Read the model definition and answer for the solid it produces. Units are mm, in the model's axes. A direction names the side the tool comes from. Give positions to 0.01 mm unless a question says otherwise; leave off trailing zeros. Write each loop counter-clockwise with the first axis right and the second up, starting at its lowest first coordinate (ties: lowest second). Pieces come first, ordered by that corner, then holes. Notation, with made-up numbers: M 60,1 L 109,1 A13 ccw 109,20 Z; hole C 70.25,-32.5 d9. An arc over 180 degrees is marked long. Put each result on its own line as item: value.
from build123d import *

# Parameters (mm, degrees)
F1_DEPTH  = 150
F2_T      = -2
F4_W      = 121
F4_H      = 42
F5_DEPTH  = 3
F6_R      = 3
F8_R      = 1.5
F8_R_2    = 0.75
F9_DEPTH  = 8.5
F10_R     = 2.5
F10_R_2   = 1.5
F12_R     = 2.5
F12_R_2   = 1.25
F13_REACH = 69.4690374315
F14_W     = 150
F14_H     = 127.2792206136
F14_W_2   = 146
F14_H_2   = 121.6223663641
F15_DEPTH = 2.5
F16_R     = 2.5
F16_R_2   = 1.25
F18_R     = 2
F19_R     = 0.5
F7_W      = 10
F7_H      = 12
F7_W_2    = 13.1
F7_H_2    = 11.7
F20_DEPTH = 3
F21_R     = 0.5
F22_R     = 0.5
F23_R     = 6.5
F24_DEPTH = 2.5
F25_R     = 2.5
F25_R_2   = 1.25
F26_DEPTH = 2.5
F27_R     = 2.5
F28_DEPTH = 1.5
F29_R     = 3


with BuildPart() as f1:
    # F0 (on Right) → F1 (new body)
    with BuildSketch(Plane.YZ):
        Polygon((63.6396103068, 63.6396103068), (0, 0), (127.2792206136, 0), align=None)
    extrude(amount=F1_DEPTH)

    # F2
    f2_openings = [f1.faces().sort_by_distance(p)[0] for p in [
        (75, 63.63961, 0),
    ]]
    offset(amount=F2_T, openings=f2_openings)

    # F4 (on offset) → F5 (cut)
    with BuildSketch(Plane(origin=(0, 0, 0), x_dir=(1, 0, 0), z_dir=(0, -0.7071067812, 0.7071067812))):
        with Locations((75, 45)):
            Rectangle(F4_W, F4_H)
    extrude(amount=-F5_DEPTH, mode=Mode.SUBTRACT)

    # F6
    f6_edges = [f1.edges().sort_by_distance(p)[0] for p in [
        (75, 63.63961, 63.63961),
    ]]
    fillet(f6_edges, radius=F6_R)

    # F8 (on face) → F9 (join)
    with BuildSketch(Plane(origin=(0, 0, 0), x_dir=(1, 0, 0), z_dir=(0, -0.7071067812, 0.7071067812))):
        with Locations((131, 67.5)):
            Circle(F8_R)
        with Locations((131, 67.5)):
            Circle(F8_R_2, mode=Mode.SUBTRACT)
        with Locations((131, 22.5)):
            Circle(F8_R)
        with Locations((131, 22.5)):
            Circle(F8_R_2, mode=Mode.SUBTRACT)
        with Locations((19, 67.5)):
            Circle(F8_R)
        with Locations((19, 67.5)):
            Circle(F8_R_2, mode=Mode.SUBTRACT)
        with Locations((19, 22.5)):
            Circle(F8_R)
        with Locations((19, 22.5)):
            Circle(F8_R_2, mode=Mode.SUBTRACT)
    extrude(amount=-F9_DEPTH)

    # F10 (on face) → F11 (join, up to the last surface of F1)
    with BuildSketch(Plane(origin=(0, 0, 0), x_dir=(1, 0, 0), z_dir=(0, 0, -1))):
        with Locations((10, -10)):
            Circle(F10_R)
        with Locations((10, -10)):
            Circle(F10_R_2, mode=Mode.SUBTRACT)
    extrude(until=Until.LAST, dir=(0, 0, 1))

    f13_end = Plane(origin=(75.2433178079, 33.3209918004, 30.4925646757), x_dir=(0, 0.7071067812, 0.7071067812), z_dir=(0, 0.7071067812, -0.7071067812))
    # F12 (on face) → F13 (join, up to a plane its end follows)
    with BuildSketch(Plane(origin=(0, 0, 0), x_dir=(1, 0, 0), z_dir=(0, 0, -1))):
        with Locations((10, -10)):
            Circle(F12_R)
        with Locations((10, -10)):
            Circle(F12_R_2, mode=Mode.SUBTRACT)
        with Locations((140, -10)):
            Circle(F12_R)
        with Locations((140, -10)):
            Circle(F12_R_2, mode=Mode.SUBTRACT)
    f13_long = extrude(amount=-F13_REACH, mode=Mode.PRIVATE)
    add(split(f13_long, bisect_by=f13_end, keep=Keep.TOP, mode=Mode.PRIVATE))

    # F14 (on face) → F15 (join)
    with BuildSketch(Plane(origin=(0, 0, 0), x_dir=(1, 0, 0), z_dir=(0, 0, -1))):
        with Locations((75, -63.6396103068)):
            Rectangle(F14_W, F14_H)
        with Locations((75, -63.6396103068)):
            Rectangle(F14_W_2, F14_H_2, mode=Mode.SUBTRACT)
    extrude(amount=F15_DEPTH)

    # F16 (on Top) → F17 (join, up to the next surface of F1)
    with BuildSketch(Plane.XY):
        with Locations((140, 117.279)):
            Circle(F16_R)
        with Locations((140, 117.279)):
            Circle(F16_R_2, mode=Mode.SUBTRACT)
        with Locations((10, 117.279)):
            Circle(F16_R)
        with Locations((10, 117.279)):
            Circle(F16_R_2, mode=Mode.SUBTRACT)
    extrude(until=Until.NEXT)

    # F18
    f18_edges = [f1.edges().sort_by_distance(p)[0] for p in [
        (150, 127.279221, -1.25),
        (150, 0, -1.25),
        (0, 0, -1.25),
        (0, 127.279221, -1.25),
    ]]
    fillet(f18_edges, radius=F18_R)

    # F19
    f19_edges = [f1.edges().sort_by_distance(p)[0] for p in [
        (0, 31.759145, 31.759145),
    ]]
    fillet(f19_edges, radius=F19_R)

    # F7 (on face) → F20 (cut)
    with BuildSketch(Plane.YZ.offset(150)):
        with Locations((95.7792206136, 10.65)):
            Rectangle(F7_W, F7_H)
        with Locations((65.3223664939, 10.0139604606)):
            Rectangle(F7_W_2, F7_H_2)
    extrude(amount=-F20_DEPTH, mode=Mode.SUBTRACT)

    # F21
    f21_edges = [f1.edges().sort_by_distance(p)[0] for p in [
        (149, 90.779221, 16.65),
        (149, 100.779221, 16.65),
    ]]
    fillet(f21_edges, radius=F21_R)

    # F22
    f22_edges = [f1.edges().sort_by_distance(p)[0] for p in [
        (149, 71.872366, 15.86396),
        (149, 58.772366, 15.86396),
    ]]
    fillet(f22_edges, radius=F22_R)

    # F23 (on face) → F24 (cut)
    with BuildSketch(Plane(origin=(0, 0, 0), x_dir=(0, -1, 0), z_dir=(-1, 0, 0))):
        with Locations((-64, 47.5)):
            Circle(F23_R)
    extrude(amount=-F24_DEPTH, mode=Mode.SUBTRACT)

    # F25 (on face) → F26 (join)
    with BuildSketch(Plane(origin=(0, 0, 0), x_dir=(1, 0, 0), z_dir=(0, 0, -1))):
        with Locations((10, -10)):
            Circle(F25_R)
        with Locations((10, -10)):
            Circle(F25_R_2, mode=Mode.SUBTRACT)
        with Locations((140, -10)):
            Circle(F25_R)
        with Locations((140, -10)):
            Circle(F25_R_2, mode=Mode.SUBTRACT)
        with Locations((10, -117.279)):
            Circle(F25_R)
        with Locations((10, -117.279)):
            Circle(F25_R_2, mode=Mode.SUBTRACT)
        with Locations((140, -117.279)):
            Circle(F25_R)
        with Locations((140, -117.279)):
            Circle(F25_R_2, mode=Mode.SUBTRACT)
    extrude(amount=F26_DEPTH)

    # F27 (on face) → F28 (cut)
    with BuildSketch(Plane(origin=(0, 0, 0), x_dir=(0, -1, 0), z_dir=(-1, 0, 0))):
        with Locations((-64, 32.5)):
            Circle(F27_R)
    extrude(amount=-F28_DEPTH, mode=Mode.SUBTRACT)

    # F29
    f29_edges = [f1.edges().sort_by_distance(p)[0] for p in [
        (75, 63.63961, 60.811183),
    ]]
    fillet(f29_edges, radius=F29_R)


solid = f1.part
(1) Which of the six approach directions +Z, -Z, +X, -X, +Y, -Y give full straight-line access (tool end or side, diameter ignored) to faces 5 (the face through (1, 58, 45)), 6 (the face through (2, 64, 15)), 7 (the face through (149.857, 32.108, 31.895))?
Result:
face 5: -X
face 6: -Z
face 7: +Z, +X, -Y
(2) Given pin 1 Ø8 at (y, z) = (64, 47.5) entering from -X; pin 2 Ø1 at (x, z) = (149.5, 13) entering from +Y; pin 3 Ø2.5 at (y, z) = (65, 32) entering from -X, each flat-ended and moving along its own axis, determine where each tip first touches the part or whether it passes through.
Result:
pin 1: stops at x = 148
pin 2: stops at y = 114.78
pin 3: stops at x = 1.5
(3) Straight lines are drawn through the part: line 1 along Y through (x, z) = (140, -2); line 2 along Z through (x, y) = (1, 64); line 3 along X through (y, z) = (27, 6). For each, find the intervals that lie inside material, in ascending order. Write a range as from..to.
Result:
line 1: y = 0..2.83, 7.5..8.75, 11.25..12.5, 114.78..116.03, 118.53..119.78, 124.45..127.28
line 2: z = -2.5..30, 35..41, 54..62.38
line 3: x = 0..2, 148..150
(4) Section A-A on x = 123 is taken. Determine the outline of the cut face in (y, z), and give its area (3 significant figures).
Result:
outline: M 0,-2.5 L 2.83,-2.5 L 2.83,0 L 18.38,15.56 L 16.97,16.97 L 0.15,0.15 A0.5 ccw 0,-0.21 Z; M 46.67,46.67 L 48.08,45.25 L 61.52,58.69 A3 cw 65.76,58.69 L 124.45,0 L 124.45,-2.5 L 127.28,-2.5 L 127.28,-0.21 A0.5 ccw 127.13,0.15 L 65.76,61.52 A3 ccw 61.52,61.52 Z
area: 282 mm²
(5) For a pull along Y with two mould halves and no side action, classify faces 1 (the face through (17.5, 19.6, 12.3)), 2 (the face through (75, 2, -2.5)), 3 (the face through (76.043, 63.607, 62.397)), 4 (the face through (0.143, 31.27, 31.057)) as +Y half, -Y half, draft (parallel to the pull), parting line (faces both ways), or undercut.
Result:
face 1: undercut
face 2: draft
face 3: parting line
face 4: -Y half
